Geometry check sheet. Reference: the model listing, model coordinates, mm. A direction names the side the tool comes from. Give positions to 0.01 mm unless a question says otherwise; leave off trailing zeros. Loops run counter-clockwise (first coordinate to the right, second up) from the corner with the lowest first, then second, coordinate; pieces in that order, holes last. Notation, with made-up numbers: (73, -26.75) -> (96, -26.75) arc R15 cw to (96, 1.25) -> close; hole circle Ø5 at (80, -29.5). An arc over 180 degrees is marked (long way). Write item = value, one per line. Start each with the question number.
```python
from build123d import *

# Parameters (mm, degrees)
SKIZZE1_W                            = 155
SKIZZE1_H                            = 140
AUFSATZ_LINEAR_AUSTRAGEN2_DEPTH      = 55
WANDUNG3_T                           = -2
SKIZZE2_W                            = 21
SKIZZE2_H                            = 24
SCHNITT_LINEAR_AUSTRAGEN1_DEPTH      = 2
SKIZZE3_R                            = 5
AUFSATZ_LINEAR_AUSTRAGEN5_DEPTH      = 25
VERRUNDUNG1_R                        = 10
F_3_0_3_DURCHMESSER_BOHRUNG1_D       = 3
F_3_0_3_DURCHMESSER_BOHRUNG1_DEPTH   = 20
F_3_0_3_DURCHMESSER_BOHRUNG1_TIP     = 0.901290929
SCHNITT_LINEAR_AUSTRAGEN2_REACH      = 119.112
SKIZZE6_W                            = 10
SKIZZE6_H                            = 10
AUFSATZ_LINEAR_AUSTRAGEN7_DEPTH      = 10
VERRUNDUNG3_R                        = 5
F_3_4_3_4_DURCHMESSER_BOHRUNG1_D     = 3.4
SKIZZE12_R                           = 5
AUFSATZ_LINEAR_AUSTRAGEN8_DEPTH      = 10
VERRUNDUNG4_R                        = 5
F_3_4_3_4_DURCHMESSER_BOHRUNG2_D     = 3.4
F_3_4_3_4_DURCHMESSER_BOHRUNG2_DEPTH = 10
F_3_4_3_4_DURCHMESSER_BOHRUNG2_TIP   = 1.021463052


with BuildPart() as part:
    # Skizze1 → Aufsatz-Linear austragen2 (new body)
    with BuildSketch(Plane.XY):
        Rectangle(SKIZZE1_W, SKIZZE1_H)
    extrude(amount=AUFSATZ_LINEAR_AUSTRAGEN2_DEPTH)

    # Wandung3
    wandung3_openings = [part.faces().sort_by_distance(p)[0] for p in [
        (0, 0, 55),
    ]]
    offset(amount=WANDUNG3_T, openings=wandung3_openings, kind=Kind.INTERSECTION)

    # Skizze2 → Schnitt-Linear austragen1 (cut)
    with BuildSketch(Plane.ZY.offset(77.5)):
        with Locations((44.5, 15)):
            Rectangle(SKIZZE2_W, SKIZZE2_H)
    extrude(amount=-SCHNITT_LINEAR_AUSTRAGEN1_DEPTH, mode=Mode.SUBTRACT)

    # Skizze3 → Aufsatz-Linear austragen5 (add)
    with BuildSketch(Plane.XY.offset(2)):
        with Locations(Location((26.111301189, -52, 0), (0, 0, 180))):
            Circle(SKIZZE3_R)
        with Locations(Location((26.111301189, 0, 0), (0, 0, 180))):
            Circle(SKIZZE3_R)
    extrude(amount=AUFSATZ_LINEAR_AUSTRAGEN5_DEPTH)

    # Verrundung1
    verrundung1_edges = [part.edges().sort_by_distance(p)[0] for p in [
        (31.111301189, -52, 2),
        (31.111301189, 0, 2),
    ]]
    fillet(verrundung1_edges, radius=VERRUNDUNG1_R)

    # Ø3.0 (3) Durchmesser Bohrung1
    with Locations(Plane.XY.offset(27)):
        with Locations((26.111301189, 0), (26.111301189, -52)):
            Hole(F_3_0_3_DURCHMESSER_BOHRUNG1_D / 2, depth=F_3_0_3_DURCHMESSER_BOHRUNG1_DEPTH)
            with Locations((0, 0, -(F_3_0_3_DURCHMESSER_BOHRUNG1_DEPTH + F_3_0_3_DURCHMESSER_BOHRUNG1_TIP / 2))):  # 118° drill point
                Cone(0, F_3_0_3_DURCHMESSER_BOHRUNG1_D / 2, F_3_0_3_DURCHMESSER_BOHRUNG1_TIP, mode=Mode.SUBTRACT)

    # Skizze6 → Schnitt-Linear austragen2 (cut, up to next)
    with BuildSketch(Plane.XY.offset(2), mode=Mode.PRIVATE) as schnitt_linear_austragen2_sk1:
        with Locations((-70.5, -63)):
            Rectangle(SKIZZE6_W, SKIZZE6_H)
    schnitt_linear_austragen2_tool1 = extrude(schnitt_linear_austragen2_sk1.sketch, amount=-SCHNITT_LINEAR_AUSTRAGEN2_REACH, mode=Mode.PRIVATE) & part.part
    # Skizze6 → Schnitt-Linear austragen2 (cut, up to next)
    with BuildSketch(Plane.XY.offset(2), mode=Mode.PRIVATE) as schnitt_linear_austragen2_sk2:
        with Locations((70.5, -63)):
            Rectangle(SKIZZE6_W, SKIZZE6_H)
    schnitt_linear_austragen2_tool2 = extrude(schnitt_linear_austragen2_sk2.sketch, amount=-SCHNITT_LINEAR_AUSTRAGEN2_REACH, mode=Mode.PRIVATE) & part.part
    # Skizze6 → Schnitt-Linear austragen2 (cut, up to next)
    with BuildSketch(Plane.XY.offset(2), mode=Mode.PRIVATE) as schnitt_linear_austragen2_sk3:
        with Locations((70.5, 63)):
            Rectangle(SKIZZE6_W, SKIZZE6_H)
    schnitt_linear_austragen2_tool3 = extrude(schnitt_linear_austragen2_sk3.sketch, amount=-SCHNITT_LINEAR_AUSTRAGEN2_REACH, mode=Mode.PRIVATE) & part.part
    # Skizze6 → Schnitt-Linear austragen2 (cut, up to next)
    with BuildSketch(Plane.XY.offset(2), mode=Mode.PRIVATE) as schnitt_linear_austragen2_sk4:
        with Locations((-70.5, 63)):
            Rectangle(SKIZZE6_W, SKIZZE6_H)
    schnitt_linear_austragen2_tool4 = extrude(schnitt_linear_austragen2_sk4.sketch, amount=-SCHNITT_LINEAR_AUSTRAGEN2_REACH, mode=Mode.PRIVATE) & part.part
    add(schnitt_linear_austragen2_tool1.solids().sort_by_distance((-70.5, -63, 2))[0], mode=Mode.SUBTRACT)
    add(schnitt_linear_austragen2_tool2.solids().sort_by_distance((70.5, -63, 2))[0], mode=Mode.SUBTRACT)
    add(schnitt_linear_austragen2_tool3.solids().sort_by_distance((70.5, 63, 2))[0], mode=Mode.SUBTRACT)
    add(schnitt_linear_austragen2_tool4.solids().sort_by_distance((-70.5, 63, 2))[0], mode=Mode.SUBTRACT)

    # 3D-Skizze1 → Aufsatz-Linear austragen7 (add)
    with BuildSketch(Plane(origin=(-75.5, 68, 47), x_dir=(0.7430494130276538, -0.6692365574288803, 0), z_dir=(0, 0, 1))):
        Polygon((0, 0), (7.43049413, 6.692365574), (14.122859705, -0.738128556), (6.692365574, -7.43049413), align=None)
        Polygon((112.200461367, 101.054720172), (104.769967237, 94.362354597), (111.462332811, 86.931860467), (118.892826941, 93.624226041), align=None)
        Polygon((203.216633178, 0), (195.786139047, -6.692365574), (189.093773473, 0.738128556), (196.524267603, 7.43049413), align=None)
        Polygon((91.01617181, -101.054720172), (98.446665941, -94.362354597), (91.754300366, -86.931860467), (84.323806236, -93.624226041), align=None)
    extrude(amount=-AUFSATZ_LINEAR_AUSTRAGEN7_DEPTH)

    # Verrundung3
    verrundung3_edges = [part.edges().sort_by_distance(p)[0] for p in [
        (-65.5, -58, 42),
        (-65.5, -68, 42),
        (-75.5, -58, 42),
        (75.5, -58, 42),
        (65.5, -58, 42),
        (65.5, -68, 42),
        (65.5, 58, 42),
        (65.5, 68, 42),
        (75.5, 58, 42),
        (-65.5, 58, 42),
        (-75.5, 58, 42),
        (-65.5, 68, 42),
    ]]
    fillet(verrundung3_edges, radius=VERRUNDUNG3_R - 0.0001)  # a hair under: the kernel refuses the full size

    # Ø3.4 (3.4) Durchmesser Bohrung1 (through all)
    with Locations(Plane.XY.offset(47)):
        with Locations((70.5, 63), (70.5, -63), (-70.5, -63), (-70.5, 63)):
            Hole(F_3_4_3_4_DURCHMESSER_BOHRUNG1_D / 2)

    # Skizze12 → Aufsatz-Linear austragen8 (add)
    with BuildSketch(Plane.XY.offset(2)):
        with Locations(Location((51.798054374, 44.186142646, 0), (0, 0, 180))):
            Circle(SKIZZE12_R)
        with Locations(Location((-8.201945626, 44.186142646, 0), (0, 0, 180))):
            Circle(SKIZZE12_R)
    extrude(amount=AUFSATZ_LINEAR_AUSTRAGEN8_DEPTH)

    # Verrundung4
    verrundung4_edges = [part.edges().sort_by_distance(p)[0] for p in [
        (56.798054374, 44.186142646, 2),
        (-3.201945626, 44.186142646, 2),
    ]]
    fillet(verrundung4_edges, radius=VERRUNDUNG4_R)

    # Ø3.4 (3.4) Durchmesser Bohrung2
    with Locations(Plane.XY.offset(12)):
        with Locations((51.798054374, 44.186142646), (-8.201945626, 44.186142646)):
            Hole(F_3_4_3_4_DURCHMESSER_BOHRUNG2_D / 2, depth=F_3_4_3_4_DURCHMESSER_BOHRUNG2_DEPTH)
            with Locations((0, 0, -(F_3_4_3_4_DURCHMESSER_BOHRUNG2_DEPTH + F_3_4_3_4_DURCHMESSER_BOHRUNG2_TIP / 2))):  # 118° drill point
                Cone(0, F_3_4_3_4_DURCHMESSER_BOHRUNG2_D / 2, F_3_4_3_4_DURCHMESSER_BOHRUNG2_TIP, mode=Mode.SUBTRACT)


solid = part.part
```
1) Depth check by flat-ended pin: pin 1 Ø12 at (x, y) = (-71, -58.5) entering from -Z; pin 2 Ø2 at (x, y) = (-76.5, 17.5) entering from +Z; pin 3 Ø11 at (x, y) = (-9.5, 45.5) entering from +Z; pin 4 Ø4.5 at (x, y) = (70.5, 61) entering from -Z. Enter the tip coordinate at first touch or a pass-through.
2) Draft check along X on faces 4 (the cylindrical face through (-68.8, -62.93, 41.93)), 5 (the flat face through (-77.5, -1, 27)). Enter one of: released by +X, released by -X, zero draft, split by the parting line, or undercut.
3) Tool access check on faces 1 (the flat face through (69, -64.4, 37)), 2 (the cylindrical face through (72.2, -62.93, 41.93)), 3 (the cylindrical face through (-64, 66.57, 41.93)). Record the directions out of +Z, -Z, +X, -X, +Y, -Y that give a thin tool (end or side, any length) a straight path to the whole face; none if there is none.
4) Thickness scan on line 1 (Y direction, x = -70.5, z = 40.5); line 2 (X direction, y = 58, z = 10); line 3 (Y direction, x = 30, z = 25). Record the ranges inside material, lowest first.
5) Section check D-D (x = -62.5). Enter the section's corners in (y, z).
6) Section check C-C (z = 41.5). Give the number of separate pieces and of enclosed holes in the cut face, plus the area to 3 significant figures.
7) Section check A-A (x = -21.5). Enter the section's corners in (y, z).
8) Section check B-B (z = 29). Enter the section's corners in (x, y).
Check result:
q1.pin_1 = 0
q1.pin_2 = 34
q1.pin_3 = 12
q1.pin_4 = 37
q2.face_4 = undercut
q2.face_5 = released by -X
q3.face_1 = none
q3.face_2 = +Z, -Z
q3.face_3 = +Z
q4.line_1 = -70 to -64.7, -61.3 to -58, 58 to 61.3, 64.7 to 70
q4.line_2 = -77.5 to -75.5, 75.5 to 77.5
q4.line_3 = -70 to -68, -55.14 to -48.86, -3.14 to 3.14, 68 to 70
q5.outline = (-70, 0) -> (70, 0) -> (70, 55) -> (68, 55) -> (68, 47) -> (67.58, 47) -> (67.58, 37) -> (68, 37) -> (68, 2) -> (-68, 2) -> (-68, 37) -> (-67.58, 37) -> (-67.58, 47) -> (-68, 47) -> (-68, 55) -> (-70, 55) -> close
q6.separate_pieces = 1
q6.enclosed_holes = 4
q6.area = 1,500 mm2
q7.outline = (-70, 0) -> (70, 0) -> (70, 55) -> (68, 55) -> (68, 2) -> (-68, 2) -> (-68, 55) -> (-70, 55) -> close
q8.outline = (-77.5, -70) -> (77.5, -70) -> (77.5, 70) -> (-77.5, 70) -> close; hole (-75.5, -68) -> (75.5, -68) -> (75.5, 68) -> (-75.5, 68) -> close
